from build123d import *

# Parameters (mm, degrees)
SKETCH1_R           = 3
BOSS_EXTRUDE1_DEPTH = 21.5
CUT_EXTRUDE1_START  = -12
CUT_EXTRUDE1_DEPTH  = 12
CHAMFER1_SIZE       = 0.5


with BuildPart() as part:
    # Sketch1 → Boss-Extrude1 (new body)
    with BuildSketch(Plane.XY):
        Circle(SKETCH1_R)
    extrude(amount=BOSS_EXTRUDE1_DEPTH)

    # Sketch2 → Cut-Extrude1 (cut)
    with BuildSketch(Plane.XY.offset(21.5).offset(CUT_EXTRUDE1_START)):
        with BuildLine():
            Line((2.5, 1.658312395), (2.5, -1.658312395))
            ThreePointArc((2.5, -1.658312395), (3, 0), (2.5, 1.658312395))
        make_face()
    extrude(amount=CUT_EXTRUDE1_DEPTH, mode=Mode.SUBTRACT)

    # Chamfer1
    chamfer1_edges = [part.edges().sort_by_distance(p)[0] for p in [
        (-3, 0, 21.5),
    ]]
    chamfer(chamfer1_edges, length=CHAMFER1_SIZE - 0.0001)  # a hair under: the kernel refuses the full size


solid = part.part
The listing builds one solid part. Answer for the finished solid, in the listing's coordinates (mm). A direction names the side the tool comes from. Coordinates: 2 decimals unless noted, no trailing zeros. Loops run counter-clockwise (first coordinate to the right, second up) from the corner with the lowest first, then second, coordinate; pieces in that order, holes last.
1) Find section A-A on z = 5.5. Write down the section's boundary in (x, y), then the cut area to 3 significant figures.
2) Find section B-B on z = 13.25. Write down the section's boundary in (x, y), then the cut area to 3 significant figures.
3) A tool of negligible diameter and unlimited length cuts with its end or side. For faces 1 (the face through (0, 0, 0)), 2 (the face through (2.5, 0, 15)), from which of +Z, -Z, +X, -X, +Y, -Y can it reach the whole face along a straight path? Write none if from no direction.
4) Flat-ended cylindrical pins translate along their axes: pin 1 Ø1 at (y, z) = (-0.5, 15) entering from +X; pin 2 Ø1 at (x, z) = (-1.5, 15) entering from +Y; pin 3 Ø1 at (x, z) = (-1.5, 15) entering from -Y. Find the tip coordinate at first contact, or state that the pin passes through.
5) Find the intervals of material crossed by L1, parallel to Y at x = 2.5, z = 6.5; L2, parallel to Z at x = 2.75, y = 0.7; L3, parallel to X at y = -0.25, z = 13.5, in increasing order.
Values:
1. outline: circle Ø6 at (0, 0)
1. area: 28.3 mm2
2. outline: (2.5, -1.66) - (2.5, 1.66) arc R3 ccw (long way) to start
2. area: 27.1 mm2
3. face 1: -Z, +X, -X, +Y, -Y
3. face 2: +Z, +X, +Y, -Y
4. pin 1: stops at x = 2.5
4. pin 2: stops at y = 2.83
4. pin 3: stops at y = -2.83
5. L1: y = -1.66 to 1.66
5. L2: z = 0 to 9.5
5. L3: x = -2.99 to 2.5
